Geometry: final body of the model. Coordinates: model frame, mm. Face numbers are marked on the shaded views. A direction names the side the tool comes from. Give positions to 0.01 mm unless a question says otherwise; leave off trailing zeros. Write each loop counter-clockwise with the first axis right and the second up, starting at its lowest first coordinate (ties: lowest second). Pieces come first, ordered by that corner, then holes. Notation, with made-up numbers: M 79.5,-9 L 134.5,-9 A21 cw 134.5,13 Z; hole C 89.5,-3.5 d2. An arc over 180 degrees is marked long. Use a Markdown table: item, result. Add a question column.
(1) Material intervals for L1, parallel to Z at x = 10, y = -95; L2, parallel to X at y = -12.5, z = 8.5; L3, parallel to Y at x = -21, z = 11.5, sorted ascending.
(2) Draft query along X for the marked faces 1, 2 and 3. Return one class per face: released by +X, released by -X, zero draft, split by the parting line, or undercut.
(3) Cut plane A-A (x = -90). Output: boundary loops of the cut face in (y, z).
(4) Pin query (flat end, axial travel): pin 1 Ø6 at (x, z) = (-12.5, 64.5) entering from -Y; pin 2 Ø4.5 at (y, z) = (-128.81, 75.94) entering from +X; pin 3 Ø3.5 at (x, z) = (-54, 157.5) entering from +Y; pin 4 Ø6.5 at (y, z) = (-119.75, 109.75) entering from -X. Return the tip coordinate at first contact, or that it passes through.
(5) Reachability of the marked faces 4 and 5 from +Z, -Z, +X, -X, +Y, -Y: full face, straight path, thin tool, end or side. Return the list, or none.
```python
from build123d import *

# Parameters (mm, degrees)
EXTRUDE_1_DEPTH          = 170
SKETCH_2_R               = 60
CUT_EXTRUDE_1_DEPTH      = 180
CUT_EXTRUDE_2_DEPTH      = 313.955268369
CUT_EXTRUDE_2_DEPTH_BACK = 313.955268369
SKETCH_3_R               = 17.5
FILLET_1_R               = 70
FILLET_2_R               = 5
FILLET_3_R               = 10
SKETCH_6_R               = 30
CUT_EXTRUDE_6_DEPTH      = 39
SKETCH_10_R              = 2.5
CUT_EXTRUDE_10_DEPTH     = 10
CUT_EXTRUDE_START        = -5.5
SKETCH_11_R              = 6
SKETCH_11_R_2            = 2.5
CUT_EXTRUDE_11_DEPTH     = 5.5
SKETCH_12_R              = 2.75
CUT_EXTRUDE_12_DEPTH     = 10
EXTRUDE_START            = 10.5
SKETCH_14_R              = 27.5
SKETCH_14_R_2            = 17.5
EXTRUDE_2_DEPTH          = 10.5
SKETCH_13_R              = 2.25
CUT_EXTRUDE_13_DEPTH     = 15
CUT_EXTRUDE_START_2      = -262
CUT_EXTRUDE_14_DEPTH     = 262
FILLET_4_R               = 10


with BuildPart() as part:
    # 草图1 → 凸台-拉伸1 (new body)
    with BuildSketch(Plane.XY):
        Polygon((-180, 0), (0, 0), (0, -175), (8, -175), (8, 8), (-180, 8), (-188, 8), (-188, -175), (-180, -175), align=None)
    extrude(amount=EXTRUDE_1_DEPTH)

    # 草图2 → 切除-拉伸1 (cut)
    with BuildSketch(Plane(origin=(0, 8, 0), x_dir=(1, 0, 0), z_dir=(0, 1, 0))):
        with Locations(Location((-90, -85, 0), (0, 0, 180))):
            Circle(SKETCH_2_R)
    extrude(amount=-CUT_EXTRUDE_1_DEPTH, mode=Mode.SUBTRACT)

    # 草图3 → 切除-拉伸2 (cut, two sides: drawn at the far end of the back side and taken through both)
    with BuildSketch(Plane(origin=(8, 0, 0), x_dir=(0, 0, -1), z_dir=(1, 0, 0)).offset(-CUT_EXTRUDE_2_DEPTH_BACK)):
        with Locations(Location((-85, -95, 0), (0, 0, 90))):
            Circle(SKETCH_3_R)
    extrude(amount=CUT_EXTRUDE_2_DEPTH + CUT_EXTRUDE_2_DEPTH_BACK, mode=Mode.SUBTRACT)

    # 圆角1
    fillet_1_edges = [part.edges().sort_by_distance(p)[0] for p in [
        (4, -175, 0),
        (4, -175, 170),
        (-184, -175, 170),
        (-184, -175, 0),
    ]]
    fillet(fillet_1_edges, radius=FILLET_1_R)

    # 圆角2
    fillet_2_edges = [part.edges().sort_by_distance(p)[0] for p in [
        (0, 0, 85),
        (-180, 0, 85),
    ]]
    fillet(fillet_2_edges, radius=FILLET_2_R)

    # 圆角3
    fillet_3_edges = [part.edges().sort_by_distance(p)[0] for p in [
        (-188, 8, 85),
        (8, 8, 85),
    ]]
    fillet(fillet_3_edges, radius=FILLET_3_R)

    # 草图6 → 切除-拉伸6 (cut)
    with BuildSketch(Plane.ZY.offset(188)):
        with Locations(Location((85, -95, 0), (0, 0, 270))):
            Circle(SKETCH_6_R)
    extrude(amount=-CUT_EXTRUDE_6_DEPTH, mode=Mode.SUBTRACT)

    # 草图10 → 切除-拉伸10 (cut)
    with BuildSketch(Plane.XZ):
        with Locations(Location((-55.742253069, 158.674753309, 0), (0, 0, 270))):
            Circle(SKETCH_10_R)
        with Locations(Location((-32.485217492, 142.390001682, 0), (0, 0, 270))):
            Circle(SKETCH_10_R)
        with Locations(Location((-9.066918551, 92.169297536, 0), (0, 0, 270))):
            Circle(SKETCH_10_R)
        with Locations(Location((-11.541409366, 63.885738097, 0), (0, 0, 270))):
            Circle(SKETCH_10_R)
        with Locations(Location((-16.325246691, 50.742253069, 0), (0, 0, 270))):
            Circle(SKETCH_10_R)
        with Locations(Location((-32.609998318, 27.485217492, 0), (0, 0, 270))):
            Circle(SKETCH_10_R)
        with Locations(Location((-124.257746931, 11.325246691, 0), (0, 0, 270))):
            Circle(SKETCH_10_R)
        with Locations(Location((-147.514782508, 27.609998318, 0), (0, 0, 270))):
            Circle(SKETCH_10_R)
        with Locations(Location((-170.933081449, 77.830702464, 0), (0, 0, 270))):
            Circle(SKETCH_10_R)
        with Locations(Location((-168.458590634, 106.114261903, 0), (0, 0, 270))):
            Circle(SKETCH_10_R)
        with Locations(Location((-163.674753309, 119.257746931, 0), (0, 0, 270))):
            Circle(SKETCH_10_R)
        with Locations(Location((-147.390001682, 142.514782508, 0), (0, 0, 270))):
            Circle(SKETCH_10_R)
    extrude(amount=-CUT_EXTRUDE_10_DEPTH, mode=Mode.SUBTRACT)

    # 草图11 → 切除-拉伸11 (cut)
    # profile 1 of 12: a face of its own
    with BuildSketch(Plane(origin=(0, 8, 0), x_dir=(1, 0, 0), z_dir=(0, 1, 0)).offset(CUT_EXTRUDE_START)):
        with Locations(Location((-32.485217492, -142.390001682, 0), (0, 0, 180))):
            Circle(SKETCH_11_R)
        with Locations(Location((-32.485217492, -142.390001682, 0), (0, 0, 90))):
            Circle(SKETCH_11_R_2, mode=Mode.SUBTRACT)
    # profile 2 of 12: a face of its own
    with BuildSketch(Plane(origin=(0, 8, 0), x_dir=(1, 0, 0), z_dir=(0, 1, 0)).offset(CUT_EXTRUDE_START)):
        with Locations(Location((-55.742253069, -158.674753309, 0), (0, 0, 180))):
            Circle(SKETCH_11_R)
        with Locations(Location((-55.742253069, -158.674753309, 0), (0, 0, 90))):
            Circle(SKETCH_11_R_2, mode=Mode.SUBTRACT)
    # profile 3 of 12: a face of its own
    with BuildSketch(Plane(origin=(0, 8, 0), x_dir=(1, 0, 0), z_dir=(0, 1, 0)).offset(CUT_EXTRUDE_START)):
        with Locations(Location((-147.390001682, -142.514782508, 0), (0, 0, 180))):
            Circle(SKETCH_11_R)
        with Locations(Location((-147.390001682, -142.514782508, 0), (0, 0, 90))):
            Circle(SKETCH_11_R_2, mode=Mode.SUBTRACT)
    # profile 4 of 12: a face of its own
    with BuildSketch(Plane(origin=(0, 8, 0), x_dir=(1, 0, 0), z_dir=(0, 1, 0)).offset(CUT_EXTRUDE_START)):
        with Locations(Location((-163.674753309, -119.257746931, 0), (0, 0, 180))):
            Circle(SKETCH_11_R)
        with Locations(Location((-163.674753309, -119.257746931, 0), (0, 0, 90))):
            Circle(SKETCH_11_R_2, mode=Mode.SUBTRACT)
    # profile 5 of 12: a face of its own
    with BuildSketch(Plane(origin=(0, 8, 0), x_dir=(1, 0, 0), z_dir=(0, 1, 0)).offset(CUT_EXTRUDE_START)):
        with Locations(Location((-168.458590634, -106.114261903, 0), (0, 0, 180))):
            Circle(SKETCH_11_R)
        with Locations(Location((-168.458590634, -106.114261903, 0), (0, 0, 90))):
            Circle(SKETCH_11_R_2, mode=Mode.SUBTRACT)
    # profile 6 of 12: a face of its own
    with BuildSketch(Plane(origin=(0, 8, 0), x_dir=(1, 0, 0), z_dir=(0, 1, 0)).offset(CUT_EXTRUDE_START)):
        with Locations(Location((-170.933081449, -77.830702464, 0), (0, 0, 180))):
            Circle(SKETCH_11_R)
        with Locations(Location((-170.933081449, -77.830702464, 0), (0, 0, 90))):
            Circle(SKETCH_11_R_2, mode=Mode.SUBTRACT)
    # profile 7 of 12: a face of its own
    with BuildSketch(Plane(origin=(0, 8, 0), x_dir=(1, 0, 0), z_dir=(0, 1, 0)).offset(CUT_EXTRUDE_START)):
        with Locations(Location((-147.514782508, -27.609998318, 0), (0, 0, 180))):
            Circle(SKETCH_11_R)
        with Locations(Location((-147.514782508, -27.609998318, 0), (0, 0, 90))):
            Circle(SKETCH_11_R_2, mode=Mode.SUBTRACT)
    # profile 8 of 12: a face of its own
    with BuildSketch(Plane(origin=(0, 8, 0), x_dir=(1, 0, 0), z_dir=(0, 1, 0)).offset(CUT_EXTRUDE_START)):
        with Locations(Location((-124.257746931, -11.325246691, 0), (0, 0, 180))):
            Circle(SKETCH_11_R)
        with Locations(Location((-124.257746931, -11.325246691, 0), (0, 0, 90))):
            Circle(SKETCH_11_R_2, mode=Mode.SUBTRACT)
    # profile 9 of 12: a face of its own
    with BuildSketch(Plane(origin=(0, 8, 0), x_dir=(1, 0, 0), z_dir=(0, 1, 0)).offset(CUT_EXTRUDE_START)):
        with Locations(Location((-32.609998318, -27.485217492, 0), (0, 0, 180))):
            Circle(SKETCH_11_R)
        with Locations(Location((-32.609998318, -27.485217492, 0), (0, 0, 90))):
            Circle(SKETCH_11_R_2, mode=Mode.SUBTRACT)
    # profile 10 of 12: a face of its own
    with BuildSketch(Plane(origin=(0, 8, 0), x_dir=(1, 0, 0), z_dir=(0, 1, 0)).offset(CUT_EXTRUDE_START)):
        with Locations(Location((-16.325246691, -50.742253069, 0), (0, 0, 180))):
            Circle(SKETCH_11_R)
        with Locations(Location((-16.325246691, -50.742253069, 0), (0, 0, 90))):
            Circle(SKETCH_11_R_2, mode=Mode.SUBTRACT)
    # profile 11 of 12: a face of its own
    with BuildSketch(Plane(origin=(0, 8, 0), x_dir=(1, 0, 0), z_dir=(0, 1, 0)).offset(CUT_EXTRUDE_START)):
        with Locations(Location((-11.541409366, -63.885738097, 0), (0, 0, 180))):
            Circle(SKETCH_11_R)
        with Locations(Location((-11.541409366, -63.885738097, 0), (0, 0, 90))):
            Circle(SKETCH_11_R_2, mode=Mode.SUBTRACT)
    # profile 12 of 12: a face of its own
    with BuildSketch(Plane(origin=(0, 8, 0), x_dir=(1, 0, 0), z_dir=(0, 1, 0)).offset(CUT_EXTRUDE_START)):
        with Locations(Location((-9.066918551, -92.169297536, 0), (0, 0, 180))):
            Circle(SKETCH_11_R)
        with Locations(Location((-9.066918551, -92.169297536, 0), (0, 0, 90))):
            Circle(SKETCH_11_R_2, mode=Mode.SUBTRACT)
    extrude(amount=CUT_EXTRUDE_11_DEPTH, mode=Mode.SUBTRACT)

    # 草图12 → 切除-拉伸12 (cut)
    with BuildSketch(Plane.ZY.offset(188)):
        with Locations(Location((94.058666579, -128.80740392, 0), (0, 0, 270))):
            Circle(SKETCH_12_R)
        with Locations(Location((75.941333421, -128.80740392, 0), (0, 0, 270))):
            Circle(SKETCH_12_R)
        with Locations(Location((60.251262658, -119.748737342, 0), (0, 0, 270))):
            Circle(SKETCH_12_R)
        with Locations(Location((51.19259608, -104.058666579, 0), (0, 0, 270))):
            Circle(SKETCH_12_R)
        with Locations(Location((51.19259608, -85.941333421, 0), (0, 0, 270))):
            Circle(SKETCH_12_R)
        with Locations(Location((60.251262658, -70.251262658, 0), (0, 0, 270))):
            Circle(SKETCH_12_R)
        with Locations(Location((75.941333421, -61.19259608, 0), (0, 0, 270))):
            Circle(SKETCH_12_R)
        with Locations(Location((94.058666579, -61.19259608, 0), (0, 0, 270))):
            Circle(SKETCH_12_R)
        with Locations(Location((109.748737342, -70.251262658, 0), (0, 0, 270))):
            Circle(SKETCH_12_R)
        with Locations(Location((118.80740392, -85.941333421, 0), (0, 0, 270))):
            Circle(SKETCH_12_R)
        with Locations(Location((118.80740392, -104.058666579, 0), (0, 0, 270))):
            Circle(SKETCH_12_R)
        with Locations(Location((109.748737342, -119.748737342, 0), (0, 0, 270))):
            Circle(SKETCH_12_R)
    extrude(amount=-CUT_EXTRUDE_12_DEPTH, mode=Mode.SUBTRACT)

    # 草图14 → 凸台-拉伸2 (add)
    with BuildSketch(Plane(origin=(8, 0, 0), x_dir=(0, 0, -1), z_dir=(1, 0, 0)).offset(EXTRUDE_START)):
        with Locations(Location((-85, -95, 0), (0, 0, 270))):
            Circle(SKETCH_14_R)
        with Locations(Location((-85, -95, 0), (0, 0, 90))):
            Circle(SKETCH_14_R_2, mode=Mode.SUBTRACT)
    extrude(amount=-EXTRUDE_2_DEPTH)

    # 草图13 → 切除-拉伸13 (cut, symmetric)
    with BuildSketch(Plane(origin=(8, 0, 0), x_dir=(0, 0, -1), z_dir=(1, 0, 0))):
        with Locations(Location((-85, -72.5, 0), (0, 0, 90))):
            Circle(SKETCH_13_R)
        with Locations(Location((-69.090097423, -79.090097423, 0), (0, 0, 90))):
            Circle(SKETCH_13_R)
        with Locations(Location((-62.5, -95, 0), (0, 0, 90))):
            Circle(SKETCH_13_R)
        with Locations(Location((-69.090097423, -110.909902577, 0), (0, 0, 90))):
            Circle(SKETCH_13_R)
        with Locations(Location((-85, -117.5, 0), (0, 0, 90))):
            Circle(SKETCH_13_R)
        with Locations(Location((-100.909902577, -110.909902577, 0), (0, 0, 90))):
            Circle(SKETCH_13_R)
        with Locations(Location((-107.5, -95, 0), (0, 0, 90))):
            Circle(SKETCH_13_R)
        with Locations(Location((-100.909902577, -79.090097423, 0), (0, 0, 90))):
            Circle(SKETCH_13_R)
    extrude(amount=CUT_EXTRUDE_13_DEPTH, both=True, mode=Mode.SUBTRACT)

    # 草图15 → 切除-拉伸14 (cut)
    with BuildSketch(Plane.ZY.offset(188).offset(CUT_EXTRUDE_START_2)):
        with BuildLine():
            Line((0, -32), (40, -32))
            Line((40, -32), (40, -95))
            ThreePointArc((40, -95), (85, -140), (130, -95))
            Line((130, -95), (130, -32))
            Line((130, -32), (170, -32))
            Line((170, -32), (170, -105))
            ThreePointArc((170, -105), (149.497474683, -154.497474683), (100, -175))
            Line((100, -175), (70, -175))
            ThreePointArc((70, -175), (20.502525317, -154.497474683), (0, -105))
            Line((0, -105), (0, -32))
        make_face()
    extrude(amount=CUT_EXTRUDE_14_DEPTH, mode=Mode.SUBTRACT)

    # 圆角4
    fillet_4_edges = [part.edges().sort_by_distance(p)[0] for p in [
        (4, -32, 40),
        (-184, -32, 40),
        (4, -32, 130),
        (-184, -32, 130),
        (4, -32, 0),
        (-184, -32, 0),
        (4, -32, 170),
        (-184, -32, 170),
    ]]
    fillet(fillet_4_edges, radius=FILLET_4_R)


solid = part.part
```
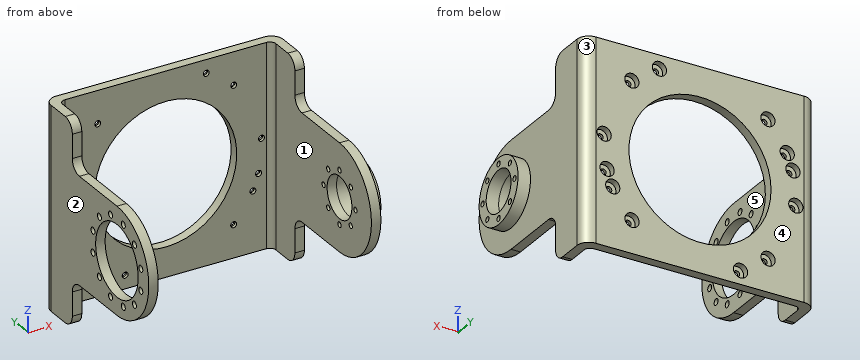
Answer list:
| question | item | result |
|---|---|---|
| 1 | L1 | 57.5 to 60.25, 64.75 to 67.5, 102.5 to 105.25, 109.75 to 112.5 |
| 1 | L2 | -188 to -180, 0 to 8 |
| 1 | L3 | 0 to 8 |
| 2 | face 1 | undercut |
| 2 | face 2 | released by -X |
| 2 | face 3 | released by +X |
| 3 | outline | M 0,0 L 8,0 L 8,25 L 0,25 Z; M 0,145 L 8,145 L 8,170 L 0,170 Z |
| 4 | pin 1 | y = 0 |
| 4 | pin 2 | x = 8 |
| 4 | pin 3 | y = 2.5 |
| 4 | pin 4 | x = -188 |
| 5 | face 4 | +Z, -Z, +X, -X, +Y |
| 5 | face 5 | +Z, -Z, -Y |
